```python
from build123d import *

# Parameters (mm, degrees)
SKETCH_1_W          = 110
SKETCH_1_H          = 115
SKETCH_1_R          = 2.25
EXTRUDE_1_DEPTH     = 2
SKETCH_2_R          = 1
SKETCH_2_R_2        = 0.5
CUT_EXTRUDE_1_DEPTH = 2
SKETCH_3_R          = 1
SKETCH_3_R_2        = 1.75
SKETCH_3_R_3        = 2.75
SKETCH_3_R_4        = 2.25
SKETCH_3_R_5        = 0.5
CUT_EXTRUDE_2_DEPTH = 2
SKETCH_4_R          = 0.5
CUT_EXTRUDE_3_DEPTH = 10


with BuildPart() as part:
    # Эскиз1 → Вытянуть1 (new body)
    with BuildSketch(Plane.XY):
        Rectangle(SKETCH_1_W, SKETCH_1_H)
        with Locations((-50, 52.5)):
            Circle(SKETCH_1_R, mode=Mode.SUBTRACT)
        with Locations(Location((50, 52.5, 0), (0, 0, 180))):
            Circle(SKETCH_1_R, mode=Mode.SUBTRACT)
        with Locations((50, -52.5)):
            Circle(SKETCH_1_R, mode=Mode.SUBTRACT)
        with Locations(Location((-50, -52.5, 0), (0, 0, 180))):
            Circle(SKETCH_1_R, mode=Mode.SUBTRACT)
    extrude(amount=EXTRUDE_1_DEPTH)

    # Эскиз2 → Вырез-Вытянуть1 (cut)
    with BuildSketch(Plane.XY.offset(2)):
        with Locations((-47.25, -37.5)):
            Circle(SKETCH_2_R)
        with Locations((-47.25, -27.5)):
            Circle(SKETCH_2_R)
        with Locations((-47.25, 26.5)):
            Circle(SKETCH_2_R)
        with Locations((-47.25, 36.5)):
            Circle(SKETCH_2_R)
        with Locations((29.55, -52.5)):
            Circle(SKETCH_2_R)
        with Locations((40.45, -52.5)):
            Circle(SKETCH_2_R)
        with Locations((-34.45, -52.5)):
            Circle(SKETCH_2_R)
        with Locations((-23.55, -52.5)):
            Circle(SKETCH_2_R)
        with Locations((-34, -44.5)):
            Circle(SKETCH_2_R_2)
        with Locations((-34, -17.5)):
            Circle(SKETCH_2_R_2)
        with Locations((-18, -44.5)):
            Circle(SKETCH_2_R_2)
        with Locations((-18, -17.5)):
            Circle(SKETCH_2_R_2)
        with Locations((-34, -47)):
            Circle(SKETCH_2_R_2)
        with Locations((-9, -49.5)):
            Circle(SKETCH_2_R)
        with Locations((1, -49.5)):
            Circle(SKETCH_2_R)
        with Locations((11, -49.5)):
            Circle(SKETCH_2_R)
        with Locations((21, -49.5)):
            Circle(SKETCH_2_R)
        with Locations((-34, -15)):
            Circle(SKETCH_2_R_2)
        with Locations((-18, -15)):
            Circle(SKETCH_2_R_2)
        with Locations((-18, -47)):
            Circle(SKETCH_2_R_2)
        with Locations((23, -35.5)):
            Circle(SKETCH_2_R_2)
        with Locations((50, -35.5)):
            Circle(SKETCH_2_R_2)
        with Locations((20.5, -35.5)):
            Circle(SKETCH_2_R_2)
        with Locations((52.5, -35.5)):
            Circle(SKETCH_2_R_2)
        with Locations((23, -25.5)):
            Circle(SKETCH_2_R_2)
        with Locations((50, -25.5)):
            Circle(SKETCH_2_R_2)
        with Locations((20.5, -25.5)):
            Circle(SKETCH_2_R_2)
        with Locations((52.5, -25.5)):
            Circle(SKETCH_2_R_2)
        with Locations((-33.5, 52.5)):
            Circle(SKETCH_2_R_2)
        with Locations((-6.5, 52.5)):
            Circle(SKETCH_2_R_2)
    extrude(amount=-CUT_EXTRUDE_1_DEPTH, mode=Mode.SUBTRACT)

    # Эскиз3 → Вырез-Вытянуть2 (cut)
    with BuildSketch(Plane.XY.offset(2)):
        with Locations((-26, 9.5)):
            Circle(SKETCH_3_R)
        with Locations((-26, -0.5)):
            Circle(SKETCH_3_R)
        with Locations((-0.5, 34.5)):
            Circle(SKETCH_3_R_2)
        with Locations((-0.5, 43.5)):
            Circle(SKETCH_3_R_3)
        with Locations((8.5, 43.5)):
            Circle(SKETCH_3_R_2)
        with Locations((8.5, 34.5)):
            Circle(SKETCH_3_R_4)
        with Locations(Location((8.5, -16.5, 0), (0, 0, 180))):
            Circle(SKETCH_3_R_2)
        with Locations(Location((8.5, -7.5, 0), (0, 0, 180))):
            Circle(SKETCH_3_R_4)
        with Locations(Location((-0.5, -16.5, 0), (0, 0, 180))):
            Circle(SKETCH_3_R_3)
        with Locations(Location((-0.5, -7.5, 0), (0, 0, 180))):
            Circle(SKETCH_3_R_2)
        with Locations((35, 12.5)):
            Circle(SKETCH_3_R)
        with Locations((35, 2.5)):
            Circle(SKETCH_3_R)
        with Locations((21, -19.5)):
            Circle(SKETCH_3_R_5)
        with Locations((18.5, -19.5)):
            Circle(SKETCH_3_R_5)
        with Locations((16, -19.5)):
            Circle(SKETCH_3_R_5)
        with Locations((21, -12.5)):
            Circle(SKETCH_3_R_5)
        with Locations((18.5, -12.5)):
            Circle(SKETCH_3_R_5)
        with Locations((16, -12.5)):
            Circle(SKETCH_3_R_5)
        with Locations((-26, -35.5)):
            Circle(SKETCH_3_R_5)
        with Locations((-26, -17.5)):
            Circle(SKETCH_3_R_5)
        with Locations((35, -43.5)):
            Circle(SKETCH_3_R_5)
        with Locations((53, -43.5)):
            Circle(SKETCH_3_R_5)
        with Locations((16, 53.5)):
            Circle(SKETCH_3_R_5)
        with Locations((34, 53.5)):
            Circle(SKETCH_3_R_5)
    extrude(amount=-CUT_EXTRUDE_2_DEPTH, mode=Mode.SUBTRACT)

    # Эскиз4 → Вырез-Вытянуть3 (cut)
    with BuildSketch(Plane.XY.offset(2)):
        with Locations((15.25, 32.5)):
            Circle(SKETCH_4_R)
        with Locations((42.75, 32.5)):
            Circle(SKETCH_4_R)
        with Locations((15.25, 44.5)):
            Circle(SKETCH_4_R)
        with Locations((42.75, 44.5)):
            Circle(SKETCH_4_R)
        with Locations((-34.75, 29.5)):
            Circle(SKETCH_4_R)
        with Locations((-7.25, 29.5)):
            Circle(SKETCH_4_R)
        with Locations((-34.75, 41.5)):
            Circle(SKETCH_4_R)
        with Locations((-7.25, 41.5)):
            Circle(SKETCH_4_R)
    extrude(amount=-CUT_EXTRUDE_3_DEPTH, mode=Mode.SUBTRACT)


solid = part.part
```
Work out the finished part from the listing and answer in its coordinate system (mm). Round coordinates to 2 decimals unless told otherwise and drop trailing zeros. Return JSON: item names as keys, results as strings. Group by question number.
Q1. The mould has two halves that part along Y. Classify faces 1 (the cylindrical face through (-2.25, 34.58, 1.01)), 2 (the flat face through (-1, 1, 2)): released by +Y, released by -Y, zero draft, split by the parting line, or undercut.
Q2. The part is cut by section A-A on z = 0.35. Count the separate pieces of the cut face and the enclosed holes in it, then the cut area to 3 significant figures.
Q3. This flat-tipped pin is pushed along its axis until it touches: pin 1 Ø1.8 at (x, y) = (40.45, -52.5) entering from +Z. Where does it stop, or does it pass through?
Q4. Find the intervals of material crossed by L1, parallel to Y at x = 23, z = 0.5; L2, parallel to X at y = -35.5, z = 0.45; L3, parallel to Y at x = -18, z = 1.45, in increasing order.
Solved:
{
 "1": {"face 1": "undercut", "face 2": "zero draft"},
 "2": {"separate pieces": "1", "enclosed holes": "66", "area": "12,400 mm²"},
 "3": {"pin 1": "through"},
 "4": {"L1": "-57.5 to -36, -35 to -26, -25 to 57.5", "L2": "-55 to -26.5, -25.5 to 20, 21 to 22.5, 23.5 to 49.5, 50.5 to 52, 53 to 55", "L3": "-57.5 to -47.5, -46.5 to -45, -44 to -18, -17 to -15.5, -14.5 to 57.5"}
}
